Job drawing, mm, ordinate dimensions from the low corner. One solid piece. A direction names the side the tool comes from. Give positions to 0.01 mm unless a question says otherwise; leave off trailing zeros. Loops run counter-clockwise (first coordinate to the right, second up) from the corner with the lowest first, then second, coordinate; pieces in that order, holes last. Notation, with made-up numbers: (24, 77) - (42, 77) arc R20 cw to (42, 85) - close; hole circle Ø5 at (-31, 83). An arc over 180 degrees is marked (long way). Answer as CSV lines item,"result". Start each with the question number.
Item 1: Saw through at B-B on x = 12.7. Give the cut face in (y, z) (3 decimals).
Item 2: Saw through at A-A on y = 39. Give the cut face in (x, z) (3 decimals), plus the area to 3 significant figures.
Item 3: Pin check, flat tip, straight feed: pin 1 (7.5 mm diameter, centred on x = 12.7, z = 9.525, fed in from +Y). Stop position of the tip, or through.
Item 4: Saw through at D-D on z = 125. Give the cut face in (x, y) (3 decimals).
Item 5: Saw through at C-C on x = 23.25. Give the cut face in (y, z) (3 decimals).
Item 6: Pull direction X, two halves, no side cores. Call the marked faces 1, 2 and 3: pulls with the +X half, pulls with the -X half, needs draft (parallel to the pull), parting line crosses it, or undercut.
Item 7: Drill centre lines: L1, parallel to Z at x = 12.7, y = 17.75 (3 decimals); L2, parallel to Z at x = 21.25, y = 39.5; L3, parallel to Z at x = 15, y = 16. Where is each one in solid material? Low to high. Write a range as from..to.
Item 8: Tool access for the marked faces 4 and 5: list every direction of +Z, -Z, +X, -X, +Y, -Y with a clear straight run to the whole face (end or side of a thin tool).
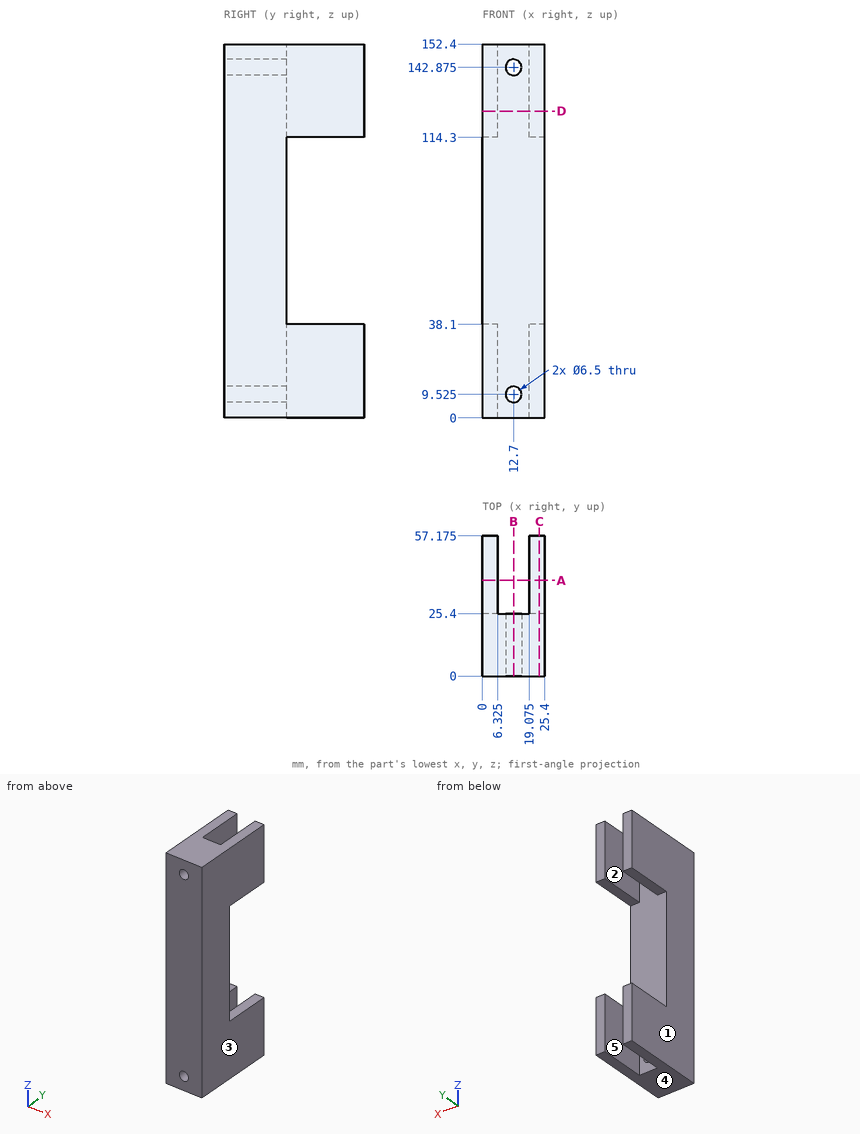
Responses:
1,outline,"(0, 0) - (25.4, 0) - (25.4, 6.275) - (0, 6.275) - close; (0, 12.775) - (25.4, 12.775) - (25.4, 139.625) - (0, 139.625) - close; (0, 146.125) - (25.4, 146.125) - (25.4, 152.4) - (0, 152.4) - close"
2,outline,"(0, 0) - (6.325, 0) - (6.325, 38.1) - (0, 38.1) - close; (0, 114.3) - (6.325, 114.3) - (6.325, 152.4) - (0, 152.4) - close; (19.075, 0) - (25.4, 0) - (25.4, 38.1) - (19.075, 38.1) - close; (19.075, 114.3) - (25.4, 114.3) - (25.4, 152.4) - (19.075, 152.4) - close"
2,area,"964 mm2"
3,pin 1,"y = 25.4"
4,outline,"(0, 0) - (25.4, 0) - (25.4, 57.175) - (19.075, 57.175) - (19.075, 25.4) - (6.325, 25.4) - (6.325, 57.175) - (0, 57.175) - close"
5,outline,"(0, 0) - (57.175, 0) - (57.175, 38.1) - (25.4, 38.1) - (25.4, 114.3) - (57.175, 114.3) - (57.175, 152.4) - (0, 152.4) - close"
6,face 1,"pulls with the -X half"
6,face 2,"undercut"
6,face 3,"pulls with the +X half"
7,L1,"0..6.275, 12.775..139.625, 146.125..152.4"
7,L2,"0..38.1, 114.3..152.4"
7,L3,"0..7.23, 11.82..140.58, 145.17..152.4"
8,face 4,"-Z, +X, -X, +Y, -Y"
8,face 5,"+Z, -Z, +Y"
